Build history of the part. All positions in model axes, mm. A direction names the side the tool comes from. Round coordinates to 2 decimals unless told otherwise and drop trailing zeros. Order: outer loops, then holes, each group sorted by start corner. A loop starts at its lowest first (then second) coordinate and runs counter-clockwise, first axis right, second up. Notation, with made-up numbers: M 74,1.5 L 110,1.5 A24 cw 110,25.5 Z; hole C 33.25,38.25 d5. An arc over 180 degrees is marked long. Use CSV: the item, a comma, the result in double quotes.
from build123d import *

# Parameters (mm, degrees)
BOSS_EXTRUDE1_DEPTH = 2


with BuildPart() as part:
    # Sketch1 → Boss-Extrude1 (new body)
    with BuildSketch(Plane(origin=(0, 0, 0), x_dir=(1, 0, 0), z_dir=(0, 1, 0))):
        with BuildLine():
            Line((0, 31.5), (0, 0))
            Line((0, 0), (71.25, 0))
            Line((71.25, 0), (71.25, 12.5))
            Line((71.25, 12.5), (16.75, 12.5))
            ThreePointArc((16.75, 12.5), (13.5, 15.75), (16.75, 19))
            Line((16.75, 19), (71.25, 19))
            Line((71.25, 19), (71.25, 31.5))
            Line((71.25, 31.5), (0, 31.5))
        make_face()
    extrude(amount=BOSS_EXTRUDE1_DEPTH)


solid = part.part
(1) Cut at B-B, the plane y = 1.1. Give the cut face in (x, z).
Answer block:
outline,"M 0,-31.5 L 71.25,-31.5 L 71.25,-19 L 16.75,-19 A3.25 cw 16.75,-12.5 L 71.25,-12.5 L 71.25,0 L 0,0 Z"
(2) Tool access for faces 1 (the face through (44, 1, -19)), 2 (the face through (71.25, 1, -6)): list every direction of +Z, -Z, +X, -X, +Y, -Y with a clear straight run to the whole face (end or side of a thin tool).
Answer block:
face 1,"+X, +Y, -Y"
face 2,"+Z, -Z, +X, +Y, -Y"
(3) Cut at C-C, the plane z = -15.75. Give the cut face in (x, y).
Answer block:
outline,"M 0,0 L 13.5,0 L 13.5,2 L 0,2 Z"
(4) Two-plate mould, pull along Z, no slides. Class faces 3 (the face through (35, 2, -12)), 4 (the face through (35, 1, 0)), 5 (the face through (44, 1, -12.5)): released by +Z, released by -Z, zero draft, split by the parting line, or undercut.
Answer block:
face 3,"zero draft"
face 4,"released by +Z"
face 5,"undercut"
(5) Wall check: line 1 (Z direction, x = 22, y = 1.45); line 2 (X direction, y = 0.75, z = -15.5); line 3 (X direction, y = 0.25, z = -18). Give the ranges that are in metal, low to high. Write a range as from..to.
Answer block:
line 1,"z = -31.5..-19, -12.5..0"
line 2,"x = 0..13.51"
line 3,"x = 0..14.4"
(6) Cut at A-A, the plane x = 41.5. Give the cut face in (y, z), and give its area (3 significant figures).
Answer block:
outline,"M 0,-31.5 L 2,-31.5 L 2,-19 L 0,-19 Z; M 0,-12.5 L 2,-12.5 L 2,0 L 0,0 Z"
area,"50.0 mm²"
